Verification items for the finished model (mm, model axes). Face numbers are marked on the shaded views. Coordinates: 2 decimals unless noted, no trailing zeros. Loops run counter-clockwise (first coordinate to the right, second up) from the corner with the lowest first, then second, coordinate; pieces in that order, holes last.
Q1. Sectioned sample at B-B (y = 0). Enter the section's corners in (x, z).
Q2. Sectioned sample at C-C (z = 25). Enter the section's corners in (x, y).
Q3. Material ranges on probe 1 along Y at (x, z) = (-21, 25); probe 2 along Y at (x, z) = (-16, 12.5); probe 3 along X at (y, z) = (-8, 42.5), recorded low to high.
Q4. Go/stop test with flat-tipped pins: P1, Ø5, axis at x = 12.5, z = 19.5, coming from the +Y side; P2, Ø1.5, axis at x = -8, z = 25, coming from the -Y side; P3, Ø6, axis at x = -4.5, z = 12.5, coming from the +Y side; P4, Ø6, axis at y = 0, z = 25, coming from the +X side. Record where each tip stops, or that it passes through.
Q5. Sectioned sample at A-A (x = 0). Enter the section's corners in (y, z).
Q6. Mould release check, pull along X, two halves, no side actions. Record for the marked faces 1, 2 and 3: +X half, -X half, draft (parallel to the pull), parting line (faces both ways), or undercut.
```python
from build123d import *

# Parameters (mm, degrees)
SKETCH1_R               = 25
BOSS_EXTRUDE1_DEPTH     = 50
SKETCH2_R               = 20
CUT_EXTRUDE1_DEPTH      = 50
CUT_EXTRUDE2_DEPTH      = 50
CUT_EXTRUDE2_DEPTH_BACK = 50
SKETCH3_R               = 2.5


with BuildPart() as part:
    # Sketch1 → Boss-Extrude1 (new body)
    with BuildSketch(Plane.XY):
        Circle(SKETCH1_R)
    extrude(amount=BOSS_EXTRUDE1_DEPTH)

    # Sketch2 → Cut-Extrude1 (cut)
    with BuildSketch(Plane.XY.offset(50)):
        Circle(SKETCH2_R)
    extrude(amount=-CUT_EXTRUDE1_DEPTH, mode=Mode.SUBTRACT)

    # Sketch3 → Cut-Extrude2 (cut, two sides: drawn at the far end of the back side and taken through both)
    with BuildSketch(Plane(origin=(0, 0, 0), x_dir=(0, 0, -1), z_dir=(1, 0, 0)).offset(-CUT_EXTRUDE2_DEPTH_BACK)):
        with Locations(Location((-25, 0, 0), (0, 0, 180))):
            Circle(SKETCH3_R)
    extrude(amount=CUT_EXTRUDE2_DEPTH + CUT_EXTRUDE2_DEPTH_BACK, mode=Mode.SUBTRACT)


solid = part.part
```
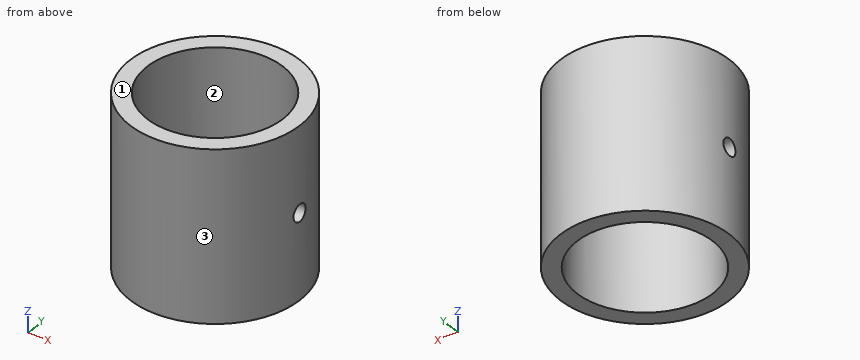
Geometry check:
1. outline: (-25, 0) - (-20, 0) - (-20, 22.5) - (-25, 22.5) - close; (-25, 27.5) - (-20, 27.5) - (-20, 50) - (-25, 50) - close; (20, 0) - (25, 0) - (25, 22.5) - (20, 22.5) - close; (20, 27.5) - (25, 27.5) - (25, 50) - (20, 50) - close
2. outline: (-24.87, -2.5) arc R25 ccw to (24.87, -2.5) - (19.84, -2.5) arc R20 cw to (-19.84, -2.5) - close; (-24.87, 2.5) - (-19.84, 2.5) arc R20 cw to (19.84, 2.5) - (24.87, 2.5) arc R25 ccw to start
3. probe 1: y = -13.56 to -2.5, 2.5 to 13.56
3. probe 2: y = -19.21 to -12, 12 to 19.21
3. probe 3: x = -23.69 to -18.33, 18.33 to 23.69
4. P1: stops at y = 22.91
4. P2: stops at y = -23.93
4. P3: stops at y = 24.95
4. P4: stops at x = 25
5. outline: (-25, 0) - (-20, 0) - (-20, 50) - (-25, 50) - close; (20, 0) - (25, 0) - (25, 50) - (20, 50) - close
6. face 1: draft
6. face 2: undercut
6. face 3: parting line
